Could you check a few things on this model? Use its own coordinates, in mm. Round coordinates to 2 decimals unless told otherwise and drop trailing zeros. Order: outer loops, then holes, each group sorted by start corner. A loop starts at its lowest first (then second) coordinate and runs counter-clockwise, first axis right, second up. Notation, with made-up numbers: (58, -27) - (67, -27) arc R14 cw to (67, -22) - close; hole circle Ø11 at (0, 89.5). An arc over 180 degrees is marked (long way). Return JSON: item names as keys, results as strings. Group by question number.
from build123d import *
from build123d.topology import SkipClean

# Parameters (mm, degrees)
SKETCH_1_R          = 1.9
EXTRUDE_1_DEPTH     = 35
SKETCH_3_R          = 1
CUT_EXTRUDE_1_DEPTH = 8
EXTRUDE_START       = 0.5
EXTRUDE_3_DEPTH     = 0.5


with BuildPart() as part:
    # 草图1 → 凸台-拉伸1 (new body)
    with BuildSketch(Plane.XY):
        Circle(SKETCH_1_R)
    extrude(amount=-EXTRUDE_1_DEPTH)

    # 草图3 → 切除-拉伸1 (cut)
    with BuildSketch(Plane.XY):
        Circle(SKETCH_3_R)
    extrude(amount=-CUT_EXTRUDE_1_DEPTH, mode=Mode.SUBTRACT)

    # 草图4 → 凸台-拉伸3 (add)
    with SkipClean():  # the faces are left unmerged after this step: merging them gives an invalid solid
        with BuildSketch(Plane.XY.offset(EXTRUDE_START)):
            with BuildLine():
                Line((-1.738533865, 0.2), (-1.889444363, 0.2))
                ThreePointArc((-1.889444363, 0.2), (-1.9, 0), (-1.889444363, -0.2))
                Line((-1.889444363, -0.2), (-1.738533865, -0.2))
                ThreePointArc((-1.738533865, -0.2), (-1.75, 0), (-1.738533865, 0.2))
            make_face()
            with BuildLine():
                ThreePointArc((1.9, 0), (1.897359256, 0.10013918), (1.889444363, 0.2))
                Line((1.889444363, 0.2), (1.738533865, 0.2))
                ThreePointArc((1.738533865, 0.2), (1.747131115, 0.100164205), (1.75, 0))
                ThreePointArc((1.75, 0), (1.747131115, -0.100164205), (1.738533865, -0.2))
                Line((1.738533865, -0.2), (1.889444363, -0.2))
                ThreePointArc((1.889444363, -0.2), (1.897359256, -0.10013918), (1.9, 0))
            make_face()
            with BuildLine():
                Line((0.2, -1.738533865), (0.2, -1.889444363))
                ThreePointArc((0.2, -1.889444363), (1.343502884, -1.343502884), (1.889444363, -0.2))
                Line((1.889444363, -0.2), (1.738533865, -0.2))
                ThreePointArc((1.738533865, -0.2), (1.237436867, -1.237436867), (0.2, -1.738533865))
            make_face()
            with BuildLine():
                Line((-0.2, -1.738533865), (-0.2, -1.889444363))
                ThreePointArc((-0.2, -1.889444363), (0, -1.9), (0.2, -1.889444363))
                Line((0.2, -1.889444363), (0.2, -1.738533865))
                ThreePointArc((0.2, -1.738533865), (0, -1.75), (-0.2, -1.738533865))
            make_face()
            with BuildLine():
                Line((-1.738533865, -0.2), (-1.889444363, -0.2))
                ThreePointArc((-1.889444363, -0.2), (-1.343502884, -1.343502884), (-0.2, -1.889444363))
                Line((-0.2, -1.889444363), (-0.2, -1.738533865))
                ThreePointArc((-0.2, -1.738533865), (-1.237436867, -1.237436867), (-1.738533865, -0.2))
            make_face()
            with BuildLine():
                ThreePointArc((-0.2, 1.889444363), (-1.343502884, 1.343502884), (-1.889444363, 0.2))
                Line((-1.889444363, 0.2), (-1.738533865, 0.2))
                ThreePointArc((-1.738533865, 0.2), (-1.237436867, 1.237436867), (-0.2, 1.738533865))
                Line((-0.2, 1.738533865), (-0.2, 1.889444363))
            make_face()
            with BuildLine():
                ThreePointArc((1.889444363, 0.2), (1.343502884, 1.343502884), (0.2, 1.889444363))
                Line((0.2, 1.889444363), (0.2, 1.738533865))
                ThreePointArc((0.2, 1.738533865), (1.237436867, 1.237436867), (1.738533865, 0.2))
                Line((1.738533865, 0.2), (1.889444363, 0.2))
            make_face()
            with BuildLine():
                ThreePointArc((0.2, 1.889444363), (0, 1.9), (-0.2, 1.889444363))
                Line((-0.2, 1.889444363), (-0.2, 1.738533865))
                ThreePointArc((-0.2, 1.738533865), (0, 1.75), (0.2, 1.738533865))
                Line((0.2, 1.738533865), (0.2, 1.889444363))
            make_face()
            with BuildLine():
                Line((-0.979795897, 0.2), (-1.738533865, 0.2))
                ThreePointArc((-1.738533865, 0.2), (-1.75, 0), (-1.738533865, -0.2))
                Line((-1.738533865, -0.2), (-0.979795897, -0.2))
                ThreePointArc((-0.979795897, -0.2), (-1, 0), (-0.979795897, 0.2))
            make_face()
            with BuildLine():
                ThreePointArc((1.75, 0), (1.747131115, 0.100164205), (1.738533865, 0.2))
                Line((1.738533865, 0.2), (0.979795897, 0.2))
                ThreePointArc((0.979795897, 0.2), (0.994936153, 0.100508962), (1, 0))
                ThreePointArc((1, 0), (0.994936153, -0.100508962), (0.979795897, -0.2))
                Line((0.979795897, -0.2), (1.738533865, -0.2))
                ThreePointArc((1.738533865, -0.2), (1.747131115, -0.100164205), (1.75, 0))
            make_face()
            with BuildLine():
                ThreePointArc((0.2, 1.738533865), (0, 1.75), (-0.2, 1.738533865))
                Line((-0.2, 1.738533865), (-0.2, 0.979795897))
                ThreePointArc((-0.2, 0.979795897), (0, 1), (0.2, 0.979795897))
                Line((0.2, 0.979795897), (0.2, 1.738533865))
            make_face()
            with BuildLine():
                Line((-0.2, -0.979795897), (-0.2, -1.738533865))
                ThreePointArc((-0.2, -1.738533865), (0, -1.75), (0.2, -1.738533865))
                Line((0.2, -1.738533865), (0.2, -0.979795897))
                ThreePointArc((0.2, -0.979795897), (0, -1), (-0.2, -0.979795897))
            make_face()
        extrude(amount=-EXTRUDE_3_DEPTH)


solid = part.part
1) If I drill on line 1 along Y through (x, z) = (0, -3.75); line 2 along X through (y, z) = (0.2, -6.5); line 3 along Z through (x, y) = (0.75, 0.75), over which ranges is the centre line in solid material (lowest first)? Write a range as from..to.
2) Will these pins go through, and if not, where does the flat tip stop? pin 1 (1 mm diameter, centred on x = -0.5, y = 0.5, fed in from +Z); pin 2 (0.6 mm diameter, centred on x = -1.5, z = 0, fed in from -Y); pin 3 (0.6 mm diameter, centred on x = 1.5, z = 0, fed in from +Y).
3) I want a section at B-B, the plane y = -1.3. List the corners of the cut face in (x, z) for me.
4) I want a section at C-C, the plane z = -23. List the corners of the cut face in (x, y) for me.
5) I want a section at A-A, the plane z = -4. List the corners of the cut face in (x, y) for me.
6) We'd pull the mould along Y, two halves only. Please class faces 1 (the flat face through (0, 0, -35)), 2 (the flat face through (0, 0, -8)): +Y half, -Y half, draft (parallel to the pull), parting line (faces both ways), or undercut.
Outcome:
{
 "1": {"line 1": "-1.9..-1, 1..1.9", "line 2": "-1.89..-0.98, 0.98..1.89", "line 3": "-35..0"},
 "2": {"pin 1": "z = 0", "pin 2": "y = -1.47", "pin 3": "y = 1.47"},
 "3": {"outline": "(-1.39, -35) - (1.39, -35) - (1.39, 0.5) - (1.17, 0.5) - (1.17, 0) - (0.2, 0) - (0.2, 0.5) - (-0.2, 0.5) - (-0.2, 0) - (-1.17, 0) - (-1.17, 0.5) - (-1.39, 0.5) - close"},
 "4": {"outline": "circle Ø3.8 at (0, 0)"},
 "5": {"outline": "circle Ø3.8 at (0, 0); hole circle Ø2 at (0, 0)"},
 "6": {"face 1": "draft", "face 2": "undercut"}
}
